Source: CAD feature listing. Evaluate the final solid. Frame: model axes, mm. A direction names the side the tool comes from. Round coordinates to 2 decimals unless told otherwise and drop trailing zeros. Loops run counter-clockwise (first coordinate to the right, second up) from the corner with the lowest first, then second, coordinate; pieces in that order, holes last.
(1) Set-up query: faces 4 (the flat face through (-31, 12.5, -29)), 5 (the flat face through (-11, 0, -30.5)). Return all of +Z, -Z, +X, -X, +Y, -Y with unobstructed straight access to the full face (end or side cutting, diameter ignored); none if empty.
(2) Mould query, pull axis Z, two halves, no side actions, for faces 1 (the flat face through (-10, 0, -32.5)), 2 (the flat face through (95.5, 0, 0)), 3 (the flat face through (97.5, 0, 0)). Classes: pulls with the +Z half, pulls with the -Z half, needs draft (parallel to the pull), parting line crosses it, or undercut.
(3) Section A-A, the plane x = -6. Return the cut outline in (y, z).
(4) First-contact query: pin 1 Ø5 at (y, z) = (-5.5, -7.5) entering from -X; pin 2 Ø0.6 at (x, y) = (-125, 2.5) entering from +Z; pin 3 Ø1.6 at (x, y) = (-125.5, -0.5) entering from -Z. Flat tips, straight axial feed; report the tip coordinate or a pass-through.
(5) Section B-B, the plane z = -6. Return the cut outline in (x, y), plus the area to 3 significant figures.
(6) Material intervals for probe 1 along Z at (x, y) = (-6.5, 4.25); probe 2 along Z at (x, y) = (40, 4); probe 3 along X at (y, z) = (8, 3.5), sorted ascending.
```python
from build123d import *
from build123d.topology import SkipClean

# Parameters (mm, degrees)
BOSS_EXTRUDE1_DEPTH = 12.5
SKETCH2_R           = 1.5
CUT_EXTRUDE1_DEPTH  = 106.770979153
BOSS_EXTRUDE2_DEPTH = 12.5
SKETCH5_W           = 219.75
SKETCH5_H           = 4
CUT_EXTRUDE4_DEPTH  = 133.741525292
CUT_EXTRUDE5_DEPTH  = 133.741525292
SKETCH7_W           = 2
SKETCH7_H           = 21.32404315
CUT_EXTRUDE6_DEPTH  = 133.741525292


with BuildPart() as part:
    # Sketch1 → Boss-Extrude1 (new, symmetric)
    with BuildSketch(Plane(origin=(0, 0, 0), x_dir=(1, 0, 0), z_dir=(0, 1, 0))):
        with BuildLine():
            Line((0, 0), (0, 32.5))
            add(Edge.make_bspline(
                [(97.5, 15), (49.867333034, 31.979096348), (0, 32.5)],
                knots=[0, 0, 0, 1, 1, 1], degree=2))
            Line((97.5, 15), (97.5, 0))
            Line((97.5, 0), (0, 0))
        make_face()
        with BuildLine():
            Line((2, 2), (2, 30.472180979))
            add(Edge.make_bspline(
                [(95.5, 13.586278965), (91.704019985, 14.92011128), (84.040035566, 17.446698519), (68.681154035, 21.845288993), (49.306403631, 26.158418674), (29.720259647, 28.881516286), (13.928614977, 30.107916443), (5.973421581, 30.403851063), (2, 30.472180979)],
                knots=[0.014029654, 0.014029654, 0.014029654, 0.014029654, 0.13472503, 0.255420406, 0.496811158, 0.73820191, 0.858897286, 0.979592662, 0.979592662, 0.979592662, 0.979592662], degree=3))
            Line((95.5, 13.586278965), (95.5, 2))
            Line((95.5, 2), (2, 2))
        make_face(mode=Mode.SUBTRACT)
    boss_extrude1 = extrude(amount=BOSS_EXTRUDE1_DEPTH, both=True)

    # Sketch2 → Cut-Extrude1 (cut, through all)
    with BuildSketch(Plane(origin=(0, 12.5, 0), x_dir=(1, 0, 0), z_dir=(0, 1, 0))):
        with Locations((0, 29)):
            Circle(SKETCH2_R)
        with Locations((94, 0)):
            Circle(SKETCH2_R)
    extrude(amount=-CUT_EXTRUDE1_DEPTH, mode=Mode.SUBTRACT)

    # Sketch3 → Boss-Extrude2 (add, symmetric)
    with BuildSketch(Plane(origin=(0, 0, 0), x_dir=(1, 0, 0), z_dir=(0, 1, 0))):
        with BuildLine():
            Line((-84.75, 0), (-71.25, 0))
            Line((-71.25, 0), (-71.25, 2))
            Line((-71.25, 2), (-86.25, 2))
            Line((-86.25, 2), (-116.25, 2))
            Line((-116.25, 2), (-124.25, 2))
            Line((-124.25, 2), (-124.25, 10.662021575))
            add(Edge.make_bspline(
                [(-124.25, 10.662021575), (-115.390155068, 11.4268576), (-97.68648523, 13.405544976), (-80.108857111, 16.28089726), (-71.325018056, 17.949728146), (-71.25, 17.96399774)],
                knots=[0.01687811, 0.01687811, 0.01687811, 0.01687811, 0.261989852, 0.507101595, 0.509213083, 0.509213083, 0.509213083, 0.509213083], degree=3))
            Line((-71.25, 17.96399774), (-71.25, 20))
            add(Edge.make_bspline(
                [(-126.25, 12.5), (-98.47520943, 14.800712755), (-71.25, 20)],
                knots=[0, 0, 0, 0.512731404, 0.512731404, 0.512731404], degree=2))
            Line((-126.25, 12.5), (-126.25, 0))
            Line((-126.25, 0), (-117.75, 0))
            ThreePointArc((-117.75, 0), (-116.25, 1.5), (-114.75, 0))
            Line((-114.75, 0), (-87.75, 0))
            ThreePointArc((-87.75, 0), (-86.25, 1.5), (-84.75, 0))
        make_face()
        with BuildLine():
            Line((-46.25, 0), (0, 0))
            Line((0, 0), (0, 27.5))
            ThreePointArc((0, 27.5), (-1.5, 29), (0, 30.5))
            Line((0, 30.5), (0, 32.5))
            Line((0, 32.5), (-20, 32.5))
            add(Edge.make_bspline(
                [(-71.25, 20), (-45.376824541, 24.941084897), (-20, 32.5)],
                knots=[0.512731404, 0.512731404, 0.512731404, 1, 1, 1], degree=2))
            Line((-71.25, 20), (-71.25, 17.96399774))
            add(Edge.make_bspline(
                [(-71.25, 17.96399774), (-62.616560883, 19.606211256), (-45.357333451, 23.34158451), (-28.233073927, 27.965983779), (-19.708743244, 30.5)],
                knots=[0.509213083, 0.509213083, 0.509213083, 0.509213083, 0.752213337, 0.99732508, 0.99732508, 0.99732508, 0.99732508], degree=3))
            Line((-19.708743244, 30.5), (-2, 30.5))
            Line((-2, 30.5), (-2, 29))
            Line((-2, 29), (-2, 27.5))
            Line((-2, 27.5), (-2, 2))
            Line((-2, 2), (-46.25, 2))
            Line((-46.25, 2), (-56.25, 2))
            Line((-56.25, 2), (-71.25, 2))
            Line((-71.25, 2), (-71.25, 0))
            Line((-71.25, 0), (-57.75, 0))
            ThreePointArc((-57.75, 0), (-56.25, 1.5), (-54.75, 0))
            Line((-54.75, 0), (-46.25, 0))
        make_face()
    boss_extrude2 = extrude(amount=BOSS_EXTRUDE2_DEPTH, both=True)

    # Mirror1: Boss-Extrude1, Boss-Extrude2 across plane
    with SkipClean():  # the faces are left unmerged after this step: merging them gives an invalid solid
        add(boss_extrude1.mirror(Plane.XY))
        add(boss_extrude2.mirror(Plane.XY))

    # Sketch5 → Cut-Extrude4 (cut, through all)
    with BuildSketch(Plane(origin=(0, 12.5, 0), x_dir=(1, 0, 0), z_dir=(0, 1, 0))):
        with Locations((-14.375, 0)):
            Rectangle(SKETCH5_W, SKETCH5_H)
    extrude(amount=-CUT_EXTRUDE4_DEPTH, mode=Mode.SUBTRACT)

    # Sketch6 → Cut-Extrude5 (cut, through all)
    with BuildSketch(Plane(origin=(0, 12.5, 0), x_dir=(1, 0, 0), z_dir=(0, 1, 0))):
        Polygon((-2, 2), (2, 2), (2, 30.472180979), (-2, 30.5), align=None)
    cut_extrude5 = extrude(amount=-CUT_EXTRUDE5_DEPTH, mode=Mode.SUBTRACT)

    # Mirror2: Cut-Extrude5 across plane
    add(cut_extrude5.mirror(Plane.XY), mode=Mode.SUBTRACT)

    # Sketch7 → Cut-Extrude6 (cut, through all)
    with BuildSketch(Plane(origin=(0, 12.5, 0), x_dir=(1, 0, 0), z_dir=(0, 1, 0))):
        with Locations((-125.25, 0)):
            Rectangle(SKETCH7_W, SKETCH7_H)
    extrude(amount=-CUT_EXTRUDE6_DEPTH, mode=Mode.SUBTRACT)


solid = part.part
```
Output values:
1. face 4: +Z, -Z, +X, -X, +Y
1. face 5: +Y, -Y
2. face 1: pulls with the -Z half
2. face 2: undercut
2. face 3: needs draft
3. outline: (-12.5, -32.5) - (12.5, -32.5) - (12.5, -30.5) - (-12.5, -30.5) - close; (-12.5, 30.5) - (12.5, 30.5) - (12.5, 32.5) - (-12.5, 32.5) - close
4. pin 1: stops at x = 95.5
4. pin 2: stops at z = 12.63
4. pin 3: stops at z = -12.63
5. outline: (95.5, -12.5) - (97.5, -12.5) - (97.5, 12.5) - (95.5, 12.5) - close
5. area: 50.0 mm2
6. probe 1: z = -32.5 to -30.5, 30.5 to 32.5
6. probe 2: z = -29.38 to -27.36, 27.36 to 29.38
6. probe 3: x = 95.5 to 97.5
